Can you work these out from the model? Positions are in its coordinate system, mm. A direction names the side the tool comes from. Round coordinates to 2 decimals unless told otherwise and drop trailing zeros. Loops run counter-clockwise (first coordinate to the right, second up) from the corner with the lowest first, then second, coordinate; pieces in that order, holes last. Notation, with made-up numbers: (23.25, 75.25) -> (36.25, 75.25) arc R23 ccw to (36.25, 110.25) -> close; hole circle Ø6 at (50.25, -9). An arc over 180 degrees is marked (long way). Write each question's results on one line, items separated by ' | '.
from build123d import *


with BuildPart() as part:
    # Sketch1 → Revolve1 (revolve)
    with BuildSketch(Plane.XY):
        with BuildLine():
            Line((-1, 0), (-7, 0))
            Line((-7, 0), (-7, -2))
            Line((-7, -2), (-9, -2))
            ThreePointArc((-9, -2), (-9.707106781, -1.707106781), (-10, -1))
            Line((-10, -1), (-10, 2))
            ThreePointArc((-10, 2), (-9.707106781, 2.707106781), (-9, 3))
            Line((-9, 3), (-1, 3))
            ThreePointArc((-1, 3), (-0.292893219, 2.707106781), (0, 2))
            Line((0, 2), (0, 1))
            ThreePointArc((0, 1), (-0.292893219, 0.292893219), (-1, 0))
        make_face()
    revolve(axis=Axis((-10, 8, 0), (1, 0, 0)))


solid = part.part
1. Will these pins go through, and if not, where does the flat tip stop? pin 1 (3 mm diameter, centred on y = 10, z = 3.5, fed in from +X); pin 2 (6 mm diameter, centred on x = -8, z = -3.5, fed in from +Y); pin 3 (5 mm diameter, centred on x = -4, y = 11, fed in from -Z).
Final values:
pin 1: x = -0.12 | pin 2: y = 17.99 | pin 3: z = -7.98
2. Please list where these lines run through material, in increasing order: line 1 (Z direction, x = -5.75, y = 8); line 2 (Y direction, x = -5, z = 0); line 3 (X direction, y = 1.5, z = 5.75). Write a range as from..to.
Final values:
line 1: -8..-5, 5..8 | line 2: 0..3, 13..16 | line 3: -10..-7
3. On a 3-axis mill with a long thin cutter (end or side, diameter ignored), from which of +Z, -Z, +X, -X, +Y, -Y can I reach the whole of each face in a straight line? I mean faces 1 (the face through (-7, 8, -8.2)), 2 (the face through (-8, 18, 0)). Say none if no direction works.
Final values:
face 1: +X | face 2: +X, -X
4. If we section it at C-C (x = -5.5): List the corners of the cut face in (y, z) for me, then the cut area to 3 significant figures.
Final values:
outline: circle Ø16 at (8, 0); hole circle Ø10 at (8, 0) | area: 123 mm2
5. If we section it at D-D (x = -8.5): List the corners of the cut face in (y, z) for me, then the cut area to 3 significant figures.
Final values:
outline: circle Ø20 at (8, 0); hole circle Ø10 at (8, 0) | area: 236 mm2
6. If we section it at A-A (y = 8): List the corners of the cut face in (x, z) for me.
Final values:
outline: (-10, -9) arc R1 ccw to (-9, -10) -> (-7, -10) -> (-7, -8) -> (-1, -8) arc R1 ccw to (0, -7) -> (0, -6) arc R1 ccw to (-1, -5) -> (-9, -5) arc R1 ccw to (-10, -6) -> close; (-10, 6) arc R1 ccw to (-9, 5) -> (-1, 5) arc R1 ccw to (0, 6) -> (0, 7) arc R1 ccw to (-1, 8) -> (-7, 8) -> (-7, 10) -> (-9, 10) arc R1 ccw to (-10, 9) -> close
7. If we section it at B-B (z = 0): List the corners of the cut face in (x, y) for me.
Final values:
outline: (-10, -1) arc R1 ccw to (-9, -2) -> (-7, -2) -> (-7, 0) -> (-1, 0) arc R1 ccw to (0, 1) -> (0, 2) arc R1 ccw to (-1, 3) -> (-9, 3) arc R1 ccw to (-10, 2) -> close; (-10, 14) arc R1 ccw to (-9, 13) -> (-1, 13) arc R1 ccw to (0, 14) -> (0, 15) arc R1 ccw to (-1, 16) -> (-7, 16) -> (-7, 18) -> (-9, 18) arc R1 ccw to (-10, 17) -> close
